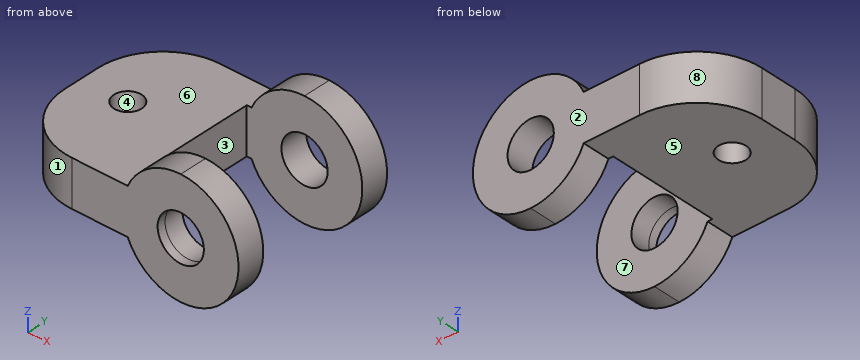
from build123d import *
from build123d.topology import SkipClean

# Parameters (mm, degrees)
CROQUIS1_R              = 1.5
SALIENTE_EXTRUIR1_DEPTH = 15
CROQUIS2_R              = 2.5
CORTAR_EXTRUIR1_DEPTH   = 20
CORTAR_EXTRUIR2_DEPTH   = 22


with BuildPart() as part:
    # Croquis1 → Saliente-Extruir1 (new body)
    with BuildSketch(Plane.XY):
        with BuildLine():
            Line((11.25, 14.1), (11.25, 11.1))
            Line((11.25, 11.1), (11.25, 5.1))
            Line((11.25, 5.1), (11.25, 2.1))
            Line((11.25, 2.1), (23.75, 2.1))
            Line((23.75, 2.1), (23.75, -0.9))
            Line((23.75, -0.9), (11.25, -0.9))
            Line((11.25, -0.9), (5.75, -0.9))
            ThreePointArc((5.75, -0.9), (0.800252532, 1.150252532), (-1.25, 6.1))
            Line((-1.25, 6.1), (-1.25, 10.1))
            ThreePointArc((-1.25, 10.1), (0.800252532, 15.049747468), (5.75, 17.1))
            Line((5.75, 17.1), (11.25, 17.1))
            Line((11.25, 17.1), (23.75, 17.1))
            Line((23.75, 17.1), (23.75, 14.1))
            Line((23.75, 14.1), (11.25, 14.1))
        make_face()
        with Locations((3.75, 8.1)):
            Circle(CROQUIS1_R, mode=Mode.SUBTRACT)
    extrude(amount=SALIENTE_EXTRUIR1_DEPTH)

    # Croquis2 → Cortar-Extruir1 (cut, symmetric)
    with BuildSketch(Plane(origin=(0, 0, 0), x_dir=(1, 0, 0), z_dir=(0, 1, 0))):
        with Locations(Location((17.5, -7.5, 0), (0, 0, 90))):
            Circle(CROQUIS2_R)
        with BuildLine():
            Line((17.5, -1.25), (11.25, 0))
            Line((11.25, 0), (11.126279301, 1.868603497))
            Line((11.126279301, 1.868603497), (29.663453957, 1.868603497))
            Line((29.663453957, 1.868603497), (29.663453957, -17.961269996))
            Line((29.663453957, -17.961269996), (11.25, -17.961269996))
            Line((11.25, -17.961269996), (11.25, -15))
            Line((11.25, -15), (17.5, -13.75))
            ThreePointArc((17.5, -13.75), (23.75, -7.5), (17.5, -1.25))
        make_face()
    extrude(amount=CORTAR_EXTRUIR1_DEPTH, both=True, mode=Mode.SUBTRACT)

    # Croquis3 → Cortar-Extruir2 (cut)
    with SkipClean():  # the faces are left unmerged after this step: merging them gives an invalid solid
        with BuildSketch(Plane(origin=(0, 17.1, 0), x_dir=(1, 0, 0), z_dir=(0, 1, 0))):
            Polygon((5.75, -10), (-2.050741432, -10), (-2.325121179, -18.2596058), (20.840368904, -18.2596058), (17.5, -13.75), (11.25, -15), (5.75, -15), align=None)
            with BuildLine():
                Line((11.771780381, -10), (5.75, -10))
                Line((5.75, -10), (5.75, -15))
                Line((5.75, -15), (11.25, -15))
                Line((11.25, -15), (17.5, -13.75))
                ThreePointArc((17.5, -13.75), (14.076734016, -12.729125166), (11.771780381, -10))
            make_face()
            with BuildLine():
                Line((5.75, 0), (5.75, -5))
                Line((5.75, -5), (11.771780381, -5))
                ThreePointArc((11.771780381, -5), (14.076734016, -2.270874834), (17.5, -1.25))
                Line((17.5, -1.25), (11.25, 0))
                Line((11.25, 0), (5.75, 0))
            make_face()
            Polygon((-2.050741432, -5), (5.75, -5), (5.75, 0), (11.25, 0), (17.5, -1.25), (17.5, 1.613327317), (-2.050741432, 1.613327317), align=None)
        extrude(amount=-CORTAR_EXTRUIR2_DEPTH, mode=Mode.SUBTRACT)


solid = part.part
Could you check a few things on this model? Use its own coordinates, in mm. Face numbers are marked on the shaded views. A direction names the side the tool comes from. Round coordinates to 2 decimals unless told otherwise and drop trailing zeros. Write each loop counter-clockwise with the first axis right and the second up, starting at its lowest first coordinate (ties: lowest second). Pieces come first, ordered by that corner, then holes. Notation, with made-up numbers: (-33, -29.5) -> (6, -29.5) arc R12 ccw to (6, -23.5) -> close; hole circle Ø11 at (-2.5, -28). An arc over 180 degrees is marked (long way). Use a Markdown table: item, result.
1. Which directions (+Z, -Z, +X, -X, +Y, -Y) give clear straight access to the entire face, cutting with the end or side of a thin tool? Please do the marked faces 4, 5, 6, 7 and 8.
Answer key:
| item | result |
|---|---|
| face 4 | +Z, -Z |
| face 5 | -Z, -X, +Y, -Y |
| face 6 | +Z, -X, +Y, -Y |
| face 7 | +Z, -Z, +X |
| face 8 | +Z, -Z, -X, +Y |
2. We'd pull the mould along Y, two halves only. Please class the marked faces 1, 2 and 3: +Y half, -Y half, draft (parallel to the pull), parting line (faces both ways), or undercut.
Answer key:
| item | result |
|---|---|
| face 1 | -Y half |
| face 2 | +Y half |
| face 3 | undercut |
3. If we section it at D-D (x = 7.25): List the corners of the cut face in (y, z) for me, then the cut area to 3 significant figures.
Answer key:
| item | result |
|---|---|
| outline | (-0.9, 5) -> (17.1, 5) -> (17.1, 10) -> (-0.9, 10) -> close |
| area | 90.0 mm^2 |
4. For pin 1 Ø4 at (x, y) = (3.75, 8.1) entering from +Z; pin 2 Ø2 at (y, z) = (12.5, 9) entering from -X; pin 3 Ø10.5 at (x, y) = (5.5, 9.5) entering from -Z, each with a flat end and sliding along its axis, tell me the tip position at first contact or that it passes through.
Answer key:
| item | result |
|---|---|
| pin 1 | stops at z = 10 |
| pin 2 | stops at x = -1.11 |
| pin 3 | stops at z = 5 |
5. If we section it at A-A (z = 7.5): List the corners of the cut face in (x, y) for me.
Answer key:
| item | result |
|---|---|
| outline | (-1.25, 6.1) arc R7 ccw to (5.75, -0.9) -> (15, -0.9) -> (15, 2.1) -> (11.25, 2.1) -> (11.25, 14.1) -> (15, 14.1) -> (15, 17.1) -> (5.75, 17.1) arc R7 ccw to (-1.25, 10.1) -> close; (20, -0.9) -> (23.75, -0.9) -> (23.75, 2.1) -> (20, 2.1) -> close; (20, 14.1) -> (23.75, 14.1) -> (23.75, 17.1) -> (20, 17.1) -> close; hole circle Ø3 at (3.75, 8.1) |
6. If we section it at C-C (z = 2.5): List the corners of the cut face in (x, y) for me, then the cut area to 3 significant figures.
Answer key:
| item | result |
|---|---|
| outline | (13.75, -0.9) -> (21.25, -0.9) -> (21.25, 2.1) -> (13.75, 2.1) -> close; (13.75, 14.1) -> (21.25, 14.1) -> (21.25, 17.1) -> (13.75, 17.1) -> close |
| area | 45.0 mm^2 |
7. If we section it at B-B (y = 8.1): List the corners of the cut face in (x, z) for me.
Answer key:
| item | result |
|---|---|
| outline | (-1.25, 5) -> (2.25, 5) -> (2.25, 10) -> (-1.25, 10) -> close; (5.25, 5) -> (11.25, 5) -> (11.25, 10) -> (5.25, 10) -> close |
8. Please list where these lines run through material, in increasing order: probe 1 along Y at (x, z) = (18, 3.75); probe 2 along Z at (x, y) = (17.5, -0.4); probe 3 along X at (y, z) = (1.5, 9).
Answer key:
| item | result |
|---|---|
| probe 1 | y = -0.9 to 2.1, 14.1 to 17.1 |
| probe 2 | z = 1.25 to 5, 10 to 13.75 |
| probe 3 | x = 0.47 to 15.5, 19.5 to 23.57 |
